Autodesk Inventor part; units mm, degrees
ref_plane "YZ Plane" through (0, 0, 0) normal (1, 0, 0) x (0, 1, 0)
ref_plane "XZ Plane" through (0, 0, 0) normal (0, 1, 0) x (-1, 0, 0)
ref_plane "XY Plane" through (0, 0, 0) normal (0, 0, 1) x (1, 0, 0)
sketch "Sketch1" plane through (0, 0, 0) normal (0, 0, 1) x (1, 0, 0)
  line L0 (-14, 44) -> (14, 44)
  line L1 (14, 44) -> (14, -44)
  line L2 (14, -44) -> (-14, -44)
  line L3 (-14, -44) -> (-14, 44)
  circle A0 centre (0, 16.5) radius 4.8
  circle A1 centre (0, -16.5) radius 4.8
  circle A2 centre (0, 36.5) radius 4.25
  circle A3 centre (0, -36.5) radius 4.25
  point P0 (0, 0)
  dimension "d0" = 28
  dimension "d2" = 9.6
  dimension "d3" = 9.6
  dimension "d8" = 8.5
  dimension "d9" = 8.5
  dimension "d11" = 20
  dimension "d12" = 20
  dimension "d37" = 44
  dimension "d38" = 44
  dimension "d45" = 33
extrude "Extrusion1" add sketch "Sketch1" along normal blind 10
sketch "Sketch2" plane through (14, -44, 0) normal (1, 0, 0) x (0, 0, -1)
  circle A0 centre (-5, 60.5) radius 1.725
  circle A1 centre (-5, 27.5) radius 1.725
  line L0 (-10, 0) -> (-10, 88)
  point P0 (0, 44)
  dimension "d23" = 3.45
  dimension "d24" = 3.45
  dimension "d25" = 16.5
  dimension "d26" = 16.5
  dimension "d27" = 5
  dimension "d28" = 5
extrude "Extrusion2" cut sketch "Sketch2" against normal blind 15
properties part number "12112_Proximal Roller Plate_V1" material "Wood (Birch)"
Geometry check sheet. Reference: the model listing, model coordinates, mm. A direction names the side the tool comes from. Coordinates: 2 decimals unless noted, no trailing zeros. Order: outer loops, then holes, each group sorted by start corner. A loop starts at its lowest first (then second) coordinate and runs counter-clockwise, first axis right, second up. Notation, with made-up numbers: (12, -39.5) - (43, -39.5) arc R28 ccw to (43, -10.5) - close; hole circle Ø3 at (0, 67.25). An arc over 180 degrees is marked (long way). Answer in a Markdown table with one row per item. Add a question column.
1) Gauge pin test, flat ends, axial feed: P1, Ø11, axis at x = 0, y = 16.5, coming from the +Z side; P2, Ø3, axis at y = -16.5, z = 5, coming from the +X side. Record the tip position at first contact, or that the pin passes through.
2) Cross-section at B-B, the plane x = 0. Record the cut outline in (y, z), then the cut area to 3 significant figures.
3) Cross-section at C-C, the plane y = 36.5. Record the cut outline in (x, z), then the cut area to 3 significant figures.
4) Material ranges on line 1 along Y through (x, z) = (0, 3.5); line 2 along Y through (x, z) = (7.75, 5) (3 decimals); line 3 along Z through (x, y) = (10.25, -16.5) (3 decimals), recorded low to high. Write a range as [from, to].
5) Release check for a two-part mould opening along Y. For faces 1 (the cylindrical face through (-4.795, 16.289, 4.93)), 2 (the flat face through (0, 44, 5)), 3 (the flat face through (14, 1, 5)) record: +Y half, -Y half, draft (parallel to the pull), parting line (faces both ways), or undercut.
6) Cross-section at D-D, the plane z = 5. Record the cut outline in (x, y) (3 decimals), then the cut area to 3 significant figures.
7) Cross-section at A-A, the plane y = -16.5. Record the cut outline in (x, z) (3 decimals), then the cut area to 3 significant figures.
8) Set-up check for faces 4 (the cylindrical face through (9.306, -18.184, 5.374)), 5 (the cylindrical face through (-4.795, -16.711, 4.93)): record each of +Z, -Z, +X, -X, +Y, -Y from which the full face is reachable in a straight line by a thin tool's end or side.
Check result:
| question | item | result |
|---|---|---|
| 1 | P1 | stops at z = 10 |
| 1 | P2 | stops at x = -4.56 |
| 2 | outline | (-44, 0) - (-40.75, 0) - (-40.75, 10) - (-44, 10) - close; (-32.25, 0) - (-21.3, 0) - (-21.3, 10) - (-32.25, 10) - close; (-11.7, 0) - (11.7, 0) - (11.7, 10) - (-11.7, 10) - close; (21.3, 0) - (32.25, 0) - (32.25, 10) - (21.3, 10) - close; (40.75, 0) - (44, 0) - (44, 10) - (40.75, 10) - close |
| 2 | area | 518 mm² |
| 3 | outline | (-14, 0) - (-4.25, 0) - (-4.25, 10) - (-14, 10) - close; (4.25, 0) - (14, 0) - (14, 10) - (4.25, 10) - close |
| 3 | area | 195 mm² |
| 4 | line 1 | y = [-44, -40.75], [-32.25, -21.3], [-11.7, 11.7], [21.3, 32.25], [40.75, 44] |
| 4 | line 2 | y = [-44, -18.225], [-14.775, 14.775], [18.225, 44] |
| 4 | line 3 | z = [0, 3.275], [6.725, 10] |
| 5 | face 1 | undercut |
| 5 | face 2 | +Y half |
| 5 | face 3 | draft |
| 6 | outline | (-14, -44) - (14, -44) - (14, -18.225) - (4.479, -18.225) arc R4.8 cw (long way) to (4.479, -14.775) - (14, -14.775) - (14, 14.775) - (4.479, 14.775) arc R4.8 cw (long way) to (4.479, 18.225) - (14, 18.225) - (14, 44) - (-14, 44) - close; hole circle Ø8.5 at (0, -36.5); hole circle Ø8.5 at (0, 36.5) |
| 6 | area | 2,140 mm² |
| 7 | outline | (-14, 0) - (-4.8, 0) - (-4.8, 10) - (-14, 10) - close; (4.8, 0) - (14, 0) - (14, 3.275) - (4.8, 3.275) - close; (4.8, 6.725) - (14, 6.725) - (14, 10) - (4.8, 10) - close |
| 7 | area | 152 mm² |
| 8 | face 4 | +X |
| 8 | face 5 | +Z, -Z |
